Verification items for the finished model (mm, model axes). Face numbers are marked on the shaded views. A direction names the side the tool comes from. Coordinates: 2 decimals unless noted, no trailing zeros. Loops run counter-clockwise (first coordinate to the right, second up) from the corner with the lowest first, then second, coordinate; pieces in that order, holes last.
Q1. Access from +Z, -Z, +X, -X, +Y, -Y to the whole of each face (thin tool, end or side, straight path). Record for the marked faces 1 and 2.
Q2. Material ranges on probe 1 along X at (y, z) = (27.5, 0); probe 2 along Y at (x, z) = (1.75, 1.5); probe 3 along Y at (x, z) = (2.75, 3), recorded low to high.
Q3. Mould release check, pull along Z, two halves, no side actions. Record for the marked faces 3, 4, 5 and 6: +Z half, -Z half, draft (parallel to the pull), parting line (faces both ways), or undercut.
Q4. Sectioned sample at A-A (y = 4). Enter the section's corners in (x, z), then the cut area to 3 significant figures.
Q5. Go/stop test with flat-tipped pins: P1, Ø3, axis at x = -1, y = -2, coming from the -Z side; P2, Ø1.5, axis at x = 1, y = 9.5, coming from the -Z side; P3, Ø6, axis at y = 6, z = 1, coming from the +X side. Record where each tip stops, or that it passes through.
```python
from build123d import *

# Parameters (mm, degrees)
SKETCH1_R           = 2
BOSS_EXTRUDE1_DEPTH = 50
BOSS_EXTRUDE2_DEPTH = 3.1
SKETCH4_R           = 1.5
BOSS_EXTRUDE3_DEPTH = 7
SKETCH5_R           = 1.5
BOSS_EXTRUDE4_DEPTH = 7


with BuildPart() as part:
    # Sketch1 → Boss-Extrude1 (new body)
    with BuildSketch(Plane(origin=(0, 0, 0), x_dir=(1, 0, 0), z_dir=(0, 1, 0))):
        with Locations(Location((0, 0, 0), (0, 0, 270))):
            Circle(SKETCH1_R)
    extrude(amount=BOSS_EXTRUDE1_DEPTH)

    # Sketch2 → Revolve1 (revolve)
    with BuildSketch(Plane.XY):
        Polygon((0, 55.6), (0, 50), (2, 50), (0.078528032, 55.6), align=None)
    revolve(axis=Axis((0, 55.6, 0), (0, -1, 0)))

    # Sketch3 → Boss-Extrude2 (add, symmetric)
    with BuildSketch(Plane(origin=(0, 0, 0), x_dir=(0, 0, -1), z_dir=(1, 0, 0))):
        Polygon((-4.2, 2.171539087), (4.2, 2.171539087), (4.029893124, -15.048329328), (-2.270106876, -15.048329328), (-5.970106876, -13.528460913), align=None)
    extrude(amount=BOSS_EXTRUDE2_DEPTH, both=True)

    # Sketch4 → Boss-Extrude3 (add)
    with BuildSketch(Plane(origin=(0, -13.673600271, 5.616776534), x_dir=(-1, 0, 0), z_dir=(0, -0.9250000000000002, 0.37996710383926635))):
        with Locations(Location((0, 1.618021252, 0), (0, 0, 270))):
            Circle(SKETCH4_R)
    extrude(amount=BOSS_EXTRUDE3_DEPTH)

    # Sketch5 → Boss-Extrude4 (add)
    with BuildSketch(Plane(origin=(0, -15.048329328, 0), x_dir=(-1, 0, 0), z_dir=(0, -1, 0))):
        with Locations(Location((0, 0.879893124, 0), (0, 0, 270))):
            Circle(SKETCH5_R)
    extrude(amount=BOSS_EXTRUDE4_DEPTH)


solid = part.part
```
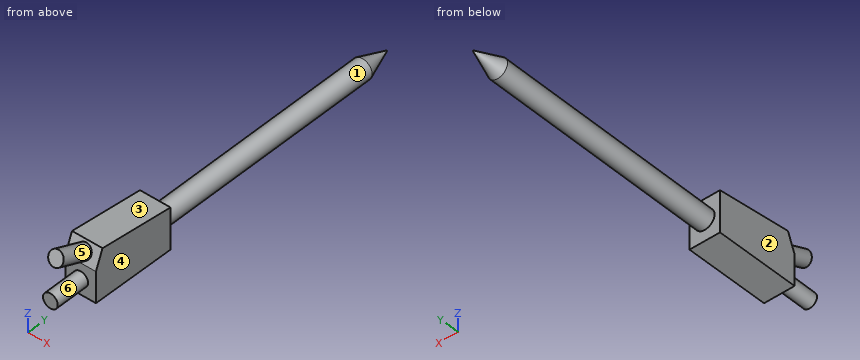
Geometry check:
1. face 1: +Y
1. face 2: +Z, -Z, -X, +Y, -Y
2. probe 1: x = -2 to 2
2. probe 2: y = -15.05 to 2.17
2. probe 3: y = -14.75 to 2.17
3. face 3: +Z half
3. face 4: draft
3. face 5: undercut
3. face 6: undercut
4. outline: circle Ø4 at (0, 0)
4. area: 12.6 mm2
5. P1: stops at z = -4.17
5. P2: stops at z = -1.98
5. P3: stops at x = 2
